Autodesk Inventor part; units mm, degrees
ref_plane "YZ Plane" through (0, 0, 0) normal (1, 0, 0) x (0, 1, 0)
ref_plane "XZ Plane" through (0, 0, 0) normal (0, 1, 0) x (-1, 0, 0)
ref_plane "XY Plane" through (0, 0, 0) normal (0, 0, 1) x (1, 0, 0)
sketch "Boceto1" plane through (0, 0, 0) normal (0, 1, 0) x (-1, 0, 0)
  line L0 (-2.031, 0) -> (-63, 0)
  line L1 (-65, -2) -> (-65, -8.0305)
  line L2 (-62.8998, -10.9676) -> (-2.0305, -10.9676)
  line L3 (0, -8.9987) -> (0, -2.031)
  line L4 (0, -8.9987) -> (0, -10.9676)
  line L5 (0, -10.9676) -> (-2.0305, -10.9676)
  line L6 (0, -2.031) -> (0, 0)
  line L7 (-65, -8.0305) -> (-65, -10.9676)
  line L8 (-65, -10.9676) -> (-62.8998, -10.9676)
  line L9 (-65, -2) -> (-65, 0)
  line L10 (-63, 0) -> (-65, 0)
  line L11 (0, 0) -> (-2.031, 0)
  dimension "d0" = 65
extrude "Extrusión1" add sketch "Boceto1" along normal blind 3
sketch "Boceto2" plane through (0, 3, 0) normal (0, 1, 0) x (1, 0, 0)
  line L0 (0, 10.9676) -> (0, 0)
  circle A0 centre (5, 5.4838) radius 2
  line L1 (65, 0) -> (65, 10.9676)
  circle A1 centre (60, 5.4838) radius 2
  line L2 (65, 5.4838) -> (60, 5.4838)
  line L3 (0, 5.4838) -> (5, 5.4838)
  point P0 (0.1384, 8.9976)
  point P1 (0.0312, 2.0308)
  point P2 (65, 2)
  point P3 (65, 8.0305)
  dimension "d20" = 5
  dimension "d31" = 4
  dimension "d32" = 4
extrude "Extrusión2" cut sketch "Boceto2" against normal blind 5
sketch "Boceto3" plane through (0, 3, 0) normal (0, 1, 0) x (1, 0, 0)
  circle A0 centre (5, 5.4838) radius 2
  line L0 (5, 5.4838) -> (319.2562, 5.4838) construction
  line L1 (19.8683, -0.0721) -> (38.3706, -22.1223)
  line L2 (16.8683, -0.0721) -> (16.8078, 0)
  line L3 (11.4418, -7.1428) -> (5.4483, 0)
  line L4 (65, 0) -> (0, 0)
  line L5 (11.4418, -7.1428) -> (29.9441, -29.1929)
  line L6 (38.3706, -22.1223) -> (29.9441, -29.1929)
  line L7 (16.8078, 0) -> (19.8078, 0)
  line L8 (0, 0) -> (65, 0)
  dimension "d37" = 3
extrude "Extrusión3" add sketch "Boceto3" against normal blind 3
sketch "Boceto10" plane through (0, 3, 0) normal (0, 1, 0) x (1, 0, 0)
  line L0 (6.3645, 0) -> (-0.0991, 7.9201)
  line L1 (-0.0991, 7.9201) -> (0, 3)
  line L2 (2.4483, 0) -> (6.3645, 0)
  line L3 (65, 0) -> (0, 0)
  line L4 (2.4483, 0) -> (0, 0)
  line L5 (0, 0) -> (0, 3)
extrude "Extrusión9" cut sketch "Boceto10" against normal blind 39
fillet "Empalme8" radius 5.48 2 edges at (65, 1.5, 0) (65, 1.5, -10.9676)
fillet "Empalme10" radius 3 2 edges at (0, 1.5, -7.7987) (0, 1.5, -10.9676)
sketch "Boceto11" plane through (0, 3, 0) normal (0, 1, 0) x (1, 0, 0)
  line L0 (0, 0) -> (0, 10.9676)
  line L1 (0, 3) -> (0, 0)
  line L2 (0, 0) -> (2.4483, 0)
  line L3 (2.4483, 0) -> (0, 3)
  line L4 (2.4483, 0) -> (0, 3)
extrude "Extrusión10" cut sketch "Boceto11" against normal blind 57.75
sketch "Boceto13" plane through (0, 3, 0) normal (0, 1, 0) x (1, 0, 0)
  arc A0 (3.7344, 10.9676) -> (1.4102, 6.0708) centre (3.7344, 7.9676) ccw
  circle A1 centre (3.7344, 7.9676) radius 1.7
  point P0 (0, 0)
  dimension "d55" = 3.4
extrude "Extrusión12" cut sketch "Boceto13" against normal blind 8
sketch "Boceto14" plane through (0, 3, 0) normal (0, 1, 0) x (1, 0, 0)
  line L0 (29.4887, -24.4468) -> (8.9754, 0)
  line L1 (59.52, 0) -> (6.3645, 0)
  line L2 (37.9152, -17.3762) -> (23.3349, 0)
  line L3 (37.9152, -17.3762) -> (29.4887, -24.4468)
  line L4 (23.3349, 0) -> (8.9754, 0)
  point P0 (0, 0)
  point P1 (37.6687, -20.1938)
  point P2 (10.2808, 0)
extrude "Extrusión18" add sketch "Boceto14" against normal blind 2
sketch "Boceto19" plane through (0, 0, 0) normal (0, -1, 0) x (1, 0, 0)
  arc A0 (59.52, -10.9676) -> (65, -5.4876) centre (59.52, -5.4876) ccw
  arc A1 (1.4102, -6.0708) -> (3.7344, -10.9676) centre (3.7344, -7.9676) ccw
  line L0 (59.52, -10.9676) -> (3.7344, -10.9676)
  line L1 (6.3645, 0) -> (1.4102, -6.0708)
  line L2 (1.4102, -6.0708) -> (6.3645, 0)
  line L3 (6.3645, 0) -> (59.52, 0)
  arc A2 (59.52, -10.9676) -> (59.52, 0) centre (59.52, -5.4838) ccw
  line L4 (3.7344, -10.9676) -> (59.52, -10.9676)
  arc A3 (1.4102, -6.0708) -> (3.7344, -10.9676) centre (3.7344, -7.9676) ccw
  circle A4 centre (60, -5.4838) radius 2
  circle A5 centre (60, -5.4838) radius 2
  circle A6 centre (3.7344, -7.9676) radius 1.7
  circle A7 centre (3.7344, -7.9676) radius 1.6
  point P0 (0, 0)
extrude "Extrusión19" cut sketch "Boceto19" against normal blind 1 contours L1 L3 A2 L0 A1
sketch "Boceto20" plane through (0, 1, 0) normal (0, -1, 0) x (1, 0, 0)
  line L0 (29.4887, 24.4468) -> (8.9754, 0)
  line L1 (1.4102, -6.0708) -> (6.3645, 0)
  line L2 (8.9754, 0) -> (1.4102, -6.0708)
  line L3 (6.3645, 0) -> (8.9754, 0)
  line L4 (8.9754, 0) -> (6, 0)
  line L5 (6, 0) -> (1.4102, -6.0708)
  point P0 (0, 0)
extrude "Extrusión20" cut sketch "Boceto20" against normal blind 11.25 contours L1 L3 L2
sketch "Boceto21" plane through (0, 1, 0) normal (0, -1, 0) x (1, 0, 0)
  line L0 (29.4887, 24.4468) -> (8.9754, 0)
  line L1 (23.3349, 0) -> (8.9754, 0)
  line L2 (16.1551, 0) -> (22.9551, 0)
  line L3 (16.1551, 0) -> (9.3551, 0)
  line L4 (22.9551, 0) -> (37.6911, 17.5642)
  line L5 (37.9152, 17.3762) -> (29.4887, 24.4468)
  line L6 (37.6911, 17.5642) -> (37.9152, 17.3762)
  line L7 (23.3349, 0) -> (59.52, 0)
  line L8 (37.9152, 17.3762) -> (23.3349, 0)
  line L9 (23.3349, 0) -> (22.9551, 0)
  line L10 (9.3551, 0) -> (8.9754, 0)
  line L11 (9.3551, 0) -> (29.7116, 24.2599)
  line L12 (29.4887, 24.4468) -> (29.7116, 24.2599)
  point P0 (0, 0)
  dimension "d89" = 6.8
  dimension "d90" = 6.8
extrude "Extrusión21" cut sketch "Boceto21" against normal blind 11.25 contours L5 L11 L1 L0 | L5 L8 L1 L4
sketch "Boceto22" plane through (0, 1, 0) normal (0, -1, 0) x (1, 0, 0)
  line L0 (37.6911, 17.5642) -> (29.7116, 24.2599)
  line L1 (29.7116, 24.2599) -> (37.6911, 17.5642)
  line L2 (37.6911, 17.5642) -> (36.0843, 15.649)
  line L3 (22.9551, 0) -> (37.6911, 17.5642)
  line L4 (36.0843, 15.649) -> (28.1043, 22.3441)
  line L5 (28.1043, 22.3441) -> (29.7116, 24.2599)
  point P0 (0, 0)
  dimension "d94" = 2.5
extrude "Extrusión22" add sketch "Boceto22" along normal blind 5
sketch "Boceto23" plane through (37.6911, -4, 17.5642) normal (0.6427876, 0, 0.7660444) x (0.7660444, 0, -0.6427876)
  line L0 (-10.4166, 7) -> (0, 7)
  line L1 (-5.2083, 7) -> (-5.2081, 0)
  line L2 (-10.4164, 0) -> (0.0002, 0)
  line L3 (0.0002, 5) -> (-10.4164, 5)
  line L4 (-5.2081, 5) -> (-5.2083, 6)
  line L5 (-5.2083, 6) -> (-5.2082, 2.6)
  circle A0 centre (-5.2082, 4.3) radius 1.7
  point P0 (-17.583, 4)
  dimension "d97" = 3.4
extrude "Extrusión23" cut sketch "Boceto23" against normal blind 10
sketch "Boceto26" plane through (0, 1, 0) normal (0, -1, 0) x (1, 0, 0)
  line L0 (33.3965, 17.904) -> (30.7918, 20.0892)
  line L1 (32.0942, 18.9966) -> (29.7959, 20.9248)
  line L2 (29.7959, 20.9248) -> (34.3925, 17.0684)
  line L3 (36.0843, 15.649) -> (33.281, 18.0009)
  line L4 (34.3925, 17.0684) -> (31.1788, 13.2379)
  line L5 (31.1788, 13.2379) -> (26.5822, 17.0943)
  line L6 (26.5822, 17.0943) -> (29.7959, 20.9248)
  point P0 (0, 0)
  point P1 (30.9074, 19.9923)
  dimension "d103" = 3
  dimension "d104" = 6
  dimension "d106" = 5
extrude "Extrusión25" cut sketch "Boceto26" against normal blind 0.9
properties part number "ventilador controladora_suportV"
Geometry: final body of the model. Coordinates: model frame, mm. A direction names the side the tool comes from. Round coordinates to 2 decimals unless told otherwise and drop trailing zeros. Order: outer loops, then holes, each group sorted by start corner. A loop starts at its lowest first (then second) coordinate and runs counter-clockwise, first axis right, second up.
Q1. Section B-B, the plane z = 7.5. Output: boundary loops of the cut face in (x, y), and give its area (3 significant figures).
Result sheet:
outline: (15.65, 1) - (29.25, 1) - (29.25, 3) - (15.65, 3) - close
area: 27.2 mm2
Q2. Mould query, pull axis X, two halves, no side actions, for faces 1 (the face through (32.81, 1.44, 15.18)), 2 (the face through (30.47, 1.44, 13.83)), 3 (the face through (63.437, 2.014, -9.32)), 4 (the face through (32, 3, -1)). Classes: released by +X, released by -X, zero draft, split by the parting line, or undercut.
Result sheet:
face 1: undercut
face 2: undercut
face 3: released by +X
face 4: zero draft
Q3. Access query for faces 5 (the face through (63.35, 2.01, -1.56)), 6 (the face through (41, 2, 0)), 7 (the face through (27.318, 1.444, 16.477)). Directions: +Z, -Z, +X, -X, +Y, -Y. A direction counts if a zero-diameter tool reaches every point of the face in a straight line with its end or side. Return the directions, or none.
Result sheet:
face 5: +Z, +X, +Y, -Y
face 6: +X, +Y, -Y
face 7: -Y
Q4. Pin query (flat end, axial travel): pin 1 (2 mm diameter, centred on x = 39.5, z = 16.5, fed in from -Y); pin 2 (6 mm diameter, centred on x = 48.5, z = -6.5, fed in from -Y); pin 3 (1.5 mm diameter, centred on y = 0, z = 19.5, fed in from +X); pin 4 (1 mm diameter, centred on x = 48.5, y = 2.5, fed in from +Z). Return the tip coordinate at first contact, or that it passes through.
Result sheet:
pin 1: passes through
pin 2: stops at y = 1
pin 3: stops at x = 36.28
pin 4: stops at z = 0
Q5. Material intervals for probe 1 along Y at (x, z) = (18, 2.5); probe 2 along Z at (x, y) = (60, 1.75); probe 3 along Y at (x, z) = (34, 19), sorted ascending.
Result sheet:
probe 1: y = 1 to 3
probe 2: z = -10.95 to -7.48, -3.48 to -0.02
probe 3: y = -4 to -0.57, 1.17 to 3
Q6. Section A-A, the plane x = 48.5. Output: boundary loops of the cut face in (y, z).
Result sheet:
outline: (1, -10.97) - (3, -10.97) - (3, 0) - (1, 0) - close
